from build123d import *

# Parameters (mm, degrees)
EXTRUSION1_DEPTH             = 48
ENL_V_MAT_EXTRU_1_DEPTH      = 97
R_P_TITION_CIRCULAIRE1_COUNT = 3
R_P_TITION_CIRCULAIRE1_ANGLE = 180


with BuildPart() as part:
    # Esquisse1 → Extrusion1 (new body, symmetric)
    with BuildSketch(Plane.XY):
        with BuildLine():
            Line((-6, 5), (-6, -5))
            ThreePointArc((-6, -5), (-5.707106781, -5.707106781), (-5, -6))
            Line((-5, -6), (5, -6))
            ThreePointArc((5, -6), (5.707106781, -5.707106781), (6, -5))
            Line((6, -5), (6, 5))
            ThreePointArc((6, 5), (5.707106781, 5.707106781), (5, 6))
            Line((5, 6), (-5, 6))
            ThreePointArc((-5, 6), (-5.707106781, 5.707106781), (-6, 5))
        make_face()
    extrude(amount=EXTRUSION1_DEPTH, both=True)

    # Esquisse3 → Enl_v. mat.-Extru.1 (cut, through all)
    with BuildSketch(Plane.XY.offset(48)):
        Polygon((6, 2), (4.8, 2), (4.8, 4), (2, 1), (2, -1), (4.8, -4), (4.8, -2), (6, -2), align=None)
    enl_v_mat_extru_1 = extrude(amount=-ENL_V_MAT_EXTRU_1_DEPTH, mode=Mode.SUBTRACT)

    # R_p_tition circulaire1: Enl_v. mat.-Extru.1 ×3 about axis
    r_p_tition_circulaire1_axis = Axis((0, 0, 0), (0, 0, 1))
    for i in range(1, R_P_TITION_CIRCULAIRE1_COUNT):
        add(enl_v_mat_extru_1.rotate(r_p_tition_circulaire1_axis, i * R_P_TITION_CIRCULAIRE1_ANGLE / (R_P_TITION_CIRCULAIRE1_COUNT - 1)), mode=Mode.SUBTRACT)


solid = part.part
Model file for the job. Use its own axes, mm. A direction names the side the tool comes from. Coordinates: 2 decimals unless noted, no trailing zeros. Write each loop counter-clockwise with the first axis right and the second up, starting at its lowest first coordinate (ties: lowest second). Pieces come first, ordered by that corner, then holes. Notation, with made-up numbers: (47.5, 34) - (73.5, 34) arc R9 cw to (73.5, 49) - close; hole circle Ø2 at (-15, -12.75). An arc over 180 degrees is marked (long way). Write each question's results on one line, items separated by ' | '. Start each with the question number.
1) Flat gauge pins, fed straight in: P1, Ø0.6, axis at x = -5.5, z = 3, coming from the +Y side; P2, Ø0.6, axis at y = 0, z = -18, coming from the -X side. Where does each tip first touch, or does it go through?
2) Probe line 1 along Y through (x, z) = (3.5, 29); line 2 along Y through (x, z) = (-3.25, 35); line 3 along X through (y, z) = (2.5, 5). List the from-to ranges inside material, lowest first. Write a range as from..to.
3) Cut at B-B (y = 0). Write the cut outline in (x, z).
4) 3-axis set-ups, long thin cutter, end or side, ignore diameter. For faces 1 (the face through (6, 3, 1)), 2 (the face through (0, 2, 1)), 3 (the face through (-2, 0, 1)), 4 (the face through (2, 0, 1)), 5 (the face through (-6, 4, 1)): which of +Z, -Z, +X, -X, +Y, -Y reach the whole face in a straight line?
5) Mould opens along Y. For faces 6 (the face through (-3.4, -2.5, 0.7)), 7 (the face through (3.4, -2.5, 0.7)), 8 (the face through (0, -6, 1)), 9 (the face through (0, -1, 48)) say: pulls with the +Y half, pulls with the -Y half, needs draft (parallel to the pull), parting line crosses it, or undercut.
Returned:
1) P1: y = 5.98 | P2: x = -2
2) line 1: -6..-2.61, 2.61..4.33, 4.8..6 | line 2: -6..-2.34, 2.34..4.1, 4.8..6 | line 3: -6..-4.8, -3.4..-1.54, 1.54..3.4, 4.8..6
3) outline: (-2, -48) - (2, -48) - (2, 48) - (-2, 48) - close
4) face 1: +Z, -Z, +X, +Y, -Y | face 2: +Z, -Z, +Y | face 3: +Z, -Z, -X | face 4: +Z, -Z, +X | face 5: +Z, -Z, -X, +Y, -Y
5) face 6: undercut | face 7: undercut | face 8: pulls with the -Y half | face 9: needs draft
